Model file for the job. Use its own axes, mm. A direction names the side the tool comes from. Round coordinates to 2 decimals unless told otherwise and drop trailing zeros. Order: outer loops, then holes, each group sorted by start corner. A loop starts at its lowest first (then second) coordinate and runs counter-clockwise, first axis right, second up. Notation, with made-up numbers: (20.5, 11.25) -> (74.5, 11.25) arc R27 ccw to (74.5, 27.25) -> close; hole circle Ø10 at (10, 10.5). An arc over 180 degrees is marked (long way). Use CSV: the item, a comma, the result in double quotes.
```python
from build123d import *

# Parameters (mm, degrees)
ESQUISSE1_R                  = 2.4
BOSS_EXTRU_1_DEPTH           = 7
ESQUISSE2_R                  = 7
BOSS_EXTRU_2_DEPTH           = 1
ESQUISSE3_R                  = 2.4
ENL_V_MAT_EXTRU_1_DEPTH      = 1
BOSS_EXTRU_3_START           = 1
ESQUISSE4_R                  = 7
BOSS_EXTRU_3_DEPTH           = 1
ENL_V_START                  = -1
ESQUISSE5_R                  = 2.4
ENL_V_MAT_EXTRU_2_DEPTH      = 1
BOSS_EXTRU_4_START           = 4
ESQUISSE6_R                  = 6.4
ESQUISSE6_R_2                = 2.4
BOSS_EXTRU_4_DEPTH           = 4
ESQUISSE7_R                  = 1.15
ENL_V_MAT_EXTRU_3_DEPTH      = 8
R_P_TITION_CIRCULAIRE1_COUNT = 3


with BuildPart() as part:
    # Esquisse1 → Boss.-Extru.1 (new body)
    with BuildSketch(Plane.XY):
        with BuildLine():
            Line((0.41669139, 5.982606575), (-0.416666667, 5.982606575))
            Line((-0.416666667, 5.982606575), (-0.416666667, 4.982608643))
            ThreePointArc((-0.416666667, 4.982608643), (-0.782160073, 4.938443644), (-1.143413046, 4.867505173))
            Line((-1.143413046, 4.867505173), (-1.452430041, 5.818561689))
            Line((-1.452430041, 5.818561689), (-2.245000651, 5.561039887))
            Line((-2.245000651, 5.561039887), (-1.935984295, 4.609985337))
            ThreePointArc((-1.935984295, 4.609985337), (-2.269941446, 4.455038253), (-2.591592247, 4.27593845))
            Line((-2.591592247, 4.27593845), (-3.179377499, 5.084955444))
            Line((-3.179377499, 5.084955444), (-3.85357833, 4.595119868))
            Line((-3.85357833, 4.595119868), (-3.265794293, 3.786104547))
            ThreePointArc((-3.265794293, 3.786104547), (-3.535525134, 3.535542677), (-3.786088342, 3.265813079))
            Line((-3.786088342, 3.265813079), (-4.595105336, 3.853598331))
            Line((-4.595105336, 3.853598331), (-5.084940912, 3.179397501))
            Line((-5.084940912, 3.179397501), (-4.27592559, 2.591613464))
            ThreePointArc((-4.27592559, 2.591613464), (-4.455026989, 2.269963551), (-4.609975731, 1.93600717))
            Line((-4.609975731, 1.93600717), (-5.561032247, 2.245024164))
            Line((-5.561032247, 2.245024164), (-5.818554049, 1.452453554))
            Line((-5.818554049, 1.452453554), (-4.867499499, 1.143437199))
            ThreePointArc((-4.867499499, 1.143437199), (-4.938439762, 0.782184577), (-4.982606575, 0.41669139))
            Line((-4.982606575, 0.41669139), (-5.982606575, 0.41669139))
            Line((-5.982606575, 0.41669139), (-5.982606575, -0.416666667))
            Line((-5.982606575, -0.416666667), (-4.982608643, -0.416666667))
            ThreePointArc((-4.982608643, -0.416666667), (-4.938443644, -0.782160073), (-4.867505173, -1.143413046))
            Line((-4.867505173, -1.143413046), (-5.818561689, -1.452430041))
            Line((-5.818561689, -1.452430041), (-5.561039887, -2.245000651))
            Line((-5.561039887, -2.245000651), (-4.609985337, -1.935984295))
            ThreePointArc((-4.609985337, -1.935984295), (-4.455038253, -2.269941446), (-4.27593845, -2.591592247))
            Line((-4.27593845, -2.591592247), (-5.084955444, -3.179377499))
            Line((-5.084955444, -3.179377499), (-4.595119868, -3.85357833))
            Line((-4.595119868, -3.85357833), (-3.786104547, -3.265794293))
            ThreePointArc((-3.786104547, -3.265794293), (-3.535542677, -3.535525134), (-3.265813079, -3.786088342))
            Line((-3.265813079, -3.786088342), (-3.853598331, -4.595105336))
            Line((-3.853598331, -4.595105336), (-3.179397501, -5.084940912))
            Line((-3.179397501, -5.084940912), (-2.591613464, -4.27592559))
            ThreePointArc((-2.591613464, -4.27592559), (-2.269963551, -4.455026989), (-1.93600717, -4.609975731))
            Line((-1.93600717, -4.609975731), (-2.245024164, -5.561032247))
            Line((-2.245024164, -5.561032247), (-1.452453554, -5.818554049))
            Line((-1.452453554, -5.818554049), (-1.143437199, -4.867499499))
            ThreePointArc((-1.143437199, -4.867499499), (-0.782184577, -4.938439762), (-0.41669139, -4.982606575))
            Line((-0.41669139, -4.982606575), (-0.41669139, -5.982606575))
            Line((-0.41669139, -5.982606575), (0.416666667, -5.982606575))
            Line((0.416666667, -5.982606575), (0.416666667, -4.982608643))
            ThreePointArc((0.416666667, -4.982608643), (0.782160073, -4.938443644), (1.143413046, -4.867505173))
            Line((1.143413046, -4.867505173), (1.452430041, -5.818561689))
            Line((1.452430041, -5.818561689), (2.245000651, -5.561039887))
            Line((2.245000651, -5.561039887), (1.935984295, -4.609985337))
            ThreePointArc((1.935984295, -4.609985337), (2.269941446, -4.455038253), (2.591592247, -4.27593845))
            Line((2.591592247, -4.27593845), (3.179377499, -5.084955444))
            Line((3.179377499, -5.084955444), (3.85357833, -4.595119868))
            Line((3.85357833, -4.595119868), (3.265794293, -3.786104547))
            ThreePointArc((3.265794293, -3.786104547), (3.535525134, -3.535542677), (3.786088342, -3.265813079))
            Line((3.786088342, -3.265813079), (4.595105336, -3.853598331))
            Line((4.595105336, -3.853598331), (5.084940912, -3.179397501))
            Line((5.084940912, -3.179397501), (4.27592559, -2.591613464))
            ThreePointArc((4.27592559, -2.591613464), (4.455026989, -2.269963551), (4.609975731, -1.93600717))
            Line((4.609975731, -1.93600717), (5.561032247, -2.245024164))
            Line((5.561032247, -2.245024164), (5.818554049, -1.452453554))
            Line((5.818554049, -1.452453554), (4.867499499, -1.143437199))
            ThreePointArc((4.867499499, -1.143437199), (4.938439762, -0.782184577), (4.982606575, -0.41669139))
            Line((4.982606575, -0.41669139), (5.982606575, -0.41669139))
            Line((5.982606575, -0.41669139), (5.982606575, 0.416666667))
            Line((5.982606575, 0.416666667), (4.982608643, 0.416666667))
            ThreePointArc((4.982608643, 0.416666667), (4.938443644, 0.782160073), (4.867505173, 1.143413046))
            Line((4.867505173, 1.143413046), (5.818561689, 1.452430041))
            Line((5.818561689, 1.452430041), (5.561039887, 2.245000651))
            Line((5.561039887, 2.245000651), (4.609985337, 1.935984295))
            ThreePointArc((4.609985337, 1.935984295), (4.455038253, 2.269941446), (4.27593845, 2.591592247))
            Line((4.27593845, 2.591592247), (5.084955444, 3.179377499))
            Line((5.084955444, 3.179377499), (4.595119868, 3.85357833))
            Line((4.595119868, 3.85357833), (3.786104547, 3.265794293))
            ThreePointArc((3.786104547, 3.265794293), (3.535542677, 3.535525134), (3.265813079, 3.786088342))
            Line((3.265813079, 3.786088342), (3.853598331, 4.595105336))
            Line((3.853598331, 4.595105336), (3.179397501, 5.084940912))
            Line((3.179397501, 5.084940912), (2.591613464, 4.27592559))
            ThreePointArc((2.591613464, 4.27592559), (2.269963551, 4.455026989), (1.93600717, 4.609975731))
            Line((1.93600717, 4.609975731), (2.245024164, 5.561032247))
            Line((2.245024164, 5.561032247), (1.452453554, 5.818554049))
            Line((1.452453554, 5.818554049), (1.143437199, 4.867499499))
            ThreePointArc((1.143437199, 4.867499499), (0.782184577, 4.938439762), (0.41669139, 4.982606575))
            Line((0.41669139, 4.982606575), (0.41669139, 5.982606575))
        make_face()
        Circle(ESQUISSE1_R, mode=Mode.SUBTRACT)
    extrude(amount=BOSS_EXTRU_1_DEPTH)

    # Esquisse2 → Boss.-Extru.2 (add)
    with BuildSketch(Plane.XY.offset(7)):
        Circle(ESQUISSE2_R)
    extrude(amount=BOSS_EXTRU_2_DEPTH)

    # Esquisse3 → Enlèv. mat.-Extru.1 (cut)
    with BuildSketch(Plane(origin=(0, 0, 7), x_dir=(-1, 0, 0), z_dir=(0, 0, -1))):
        Circle(ESQUISSE3_R)
    extrude(amount=-ENL_V_MAT_EXTRU_1_DEPTH, mode=Mode.SUBTRACT)

    # Esquisse4 → Boss.-Extru.3 (add)
    with BuildSketch(Plane(origin=(0, 0, 0), x_dir=(-1, 0, 0), z_dir=(0, 0, -1)).offset(BOSS_EXTRU_3_START)):
        with Locations(Location((0, 0, 0), (0, 0, 180))):
            Circle(ESQUISSE4_R)
    extrude(amount=-BOSS_EXTRU_3_DEPTH)

    # Esquisse5 → Enlèv. mat.-Extru.2 (cut)
    with BuildSketch(Plane.XY.offset(ENL_V_START)):
        with Locations(Location((0, 0, 0), (0, 0, 180))):
            Circle(ESQUISSE5_R)
    extrude(amount=ENL_V_MAT_EXTRU_2_DEPTH, mode=Mode.SUBTRACT)

    # Esquisse6 → Boss.-Extru.4 (add)
    with BuildSketch(Plane(origin=(0, 0, -1), x_dir=(-1, 0, 0), z_dir=(0, 0, -1)).offset(BOSS_EXTRU_4_START)):
        Circle(ESQUISSE6_R)
        Circle(ESQUISSE6_R_2, mode=Mode.SUBTRACT)
    extrude(amount=-BOSS_EXTRU_4_DEPTH)

    # Esquisse7 → Enlèv. mat.-Extru.3 (cut)
    with BuildSketch(Plane(origin=(0, 0, 0), x_dir=(0, 0, -1), z_dir=(1, 0, 0))):
        with Locations((3, 0)):
            Circle(ESQUISSE7_R)
    enl_v_mat_extru_3 = extrude(amount=-ENL_V_MAT_EXTRU_3_DEPTH, mode=Mode.SUBTRACT)

    # Répétition circulaire1: Enlèv. mat.-Extru.3 ×3 about axis
    r_p_tition_circulaire1_axis = Axis((0, 0, 0), (0, 0, -1))
    for i in range(1, R_P_TITION_CIRCULAIRE1_COUNT):
        add(enl_v_mat_extru_3.rotate(r_p_tition_circulaire1_axis, i * 360 / R_P_TITION_CIRCULAIRE1_COUNT), mode=Mode.SUBTRACT)


solid = part.part
```
Q1. Cut at A-A (z = -3). Give the cut face in (x, y).
From the geometry:
outline,"(-6.3, -1.15) arc R6.4 ccw to (2.15, -6.03) -> (0.06, -2.4) arc R2.4 cw to (-2.11, -1.15) -> close; (-6.3, 1.15) -> (-2.11, 1.15) arc R2.4 cw to (0.06, 2.4) -> (2.15, 6.03) arc R6.4 ccw to start; (2.05, -1.25) -> (4.14, -4.88) arc R6.4 ccw to (4.14, 4.88) -> (2.05, 1.25) arc R2.4 cw to start"
Q2. Cut at B-B (y = 0). Give the cut face in (x, z).
From the geometry:
outline,"(-7, -1) -> (-6.4, -1) -> (-6.4, -1.85) -> (-2.4, -1.85) -> (-2.4, 8) -> (-7, 8) -> (-7, 7) -> (-5.98, 7) -> (-5.98, 0) -> (-7, 0) -> close; (-6.4, -5) -> (-2.4, -5) -> (-2.4, -4.15) -> (-6.4, -4.15) -> close; (2.4, -5) -> (6.4, -5) -> (6.4, -1) -> (7, -1) -> (7, 0) -> (5.98, 0) -> (5.98, 7) -> (7, 7) -> (7, 8) -> (2.4, 8) -> close"
Q3. Cut at C-C (z = -0.25). Give the cut face in (x, y).
From the geometry:
outline,"circle Ø14 at (0, 0); hole circle Ø4.8 at (0, 0)"
Q4. Which spindle directions (+Z, -Z, +X, -X, +Y, -Y) get a long thin tool onto all of the face, cutting with end or side? Do faces 1 (the flat face through (-4, -4, 0)), 2 (the flat face through (-5.35, 1.3, 3.45)), 3 (the flat face through (4.7, 2.9, 3.5)), 4 (the flat face through (-2.9, 4.7, 3.5)). Say none if no direction does.
From the geometry:
face 1,"none"
face 2,"-X"
face 3,"+X"
face 4,"+Y"
Q5. Mould opens along Y. For faces 5 (the flat face through (-1.296, 5.336, 3.451)), 6 (the flat face through (-0.417, -5.5, 3.5)), 7 (the flat face through (-5.336, -1.296, 3.451)) say: +Y half, -Y half, draft (parallel to the pull), parting line (faces both ways), or undercut.
From the geometry:
face 5,"+Y half"
face 6,"draft"
face 7,"undercut"
Q6. Pin check, flat tips, straight feed: pin 1 (5 mm diameter, centred on x = 4, z = -3.5, fed in from +Y); pin 2 (1.8 mm diameter, centred on y = 0, z = -3, fed in from +X); pin 3 (0.5 mm diameter, centred on x = -5.5, z = 3.5, fed in from -Y) (3 decimals); pin 4 (4 mm diameter, centred on x = 0, y = 0, fed in from -Z). Stop position of each tip, or through.
From the geometry:
pin 1,"stops at y = 6.22"
pin 2,"stops at x = 6.4"
pin 3,"stops at y = -2.245"
pin 4,"passes through"
Q7. Probe line 1 along Y through (x, z) = (0, 4.75); line 2 along Z through (x, y) = (-5.5, 0); line 3 along Y through (x, z) = (0, -3.05). List the from-to ranges inside material, lowest first.
From the geometry:
line 1,"y = -5.98 to -2.4, 2.4 to 5.98"
line 2,"z = -5 to -4.15, -1.85 to 8"
line 3,"y = -6.4 to -2.4, 2.4 to 6.4"
Q8. Cut at D-D (x = 3.5). State how many separate pieces and enclosed holes the cut face has, plus the area to 3 significant figures.
From the geometry:
separate pieces,"1"
enclosed holes,"2"
area,"122 mm²"
